```python
from build123d import *

# Parameters (mm, degrees)
F0_R     = 1.0414
F1_DEPTH = 12.7
F3_DEPTH = 25.4
F5_D     = 2.0828
F7_D     = 2.0828
F7_DEPTH = 15.24
F7_TIP   = 0.6257362487


with BuildPart() as f1:
    # F0 (on Top) → F1 (new body)
    with BuildSketch(Plane.XY):
        with BuildLine():
            ThreePointArc((-68.834, -11.2141), (-67.3461024484, -14.8062024484), (-63.754, -16.2941))
            Line((-63.754, -16.2941), (63.754, -16.2941))
            ThreePointArc((63.754, -16.2941), (67.3461024484, -14.8062024484), (68.834, -11.2141))
            Line((68.834, -11.2141), (68.834, 11.2141))
            ThreePointArc((68.834, 11.2141), (67.3461024484, 14.8062024484), (63.754, 16.2941))
            Line((63.754, 16.2941), (-63.754, 16.2941))
            ThreePointArc((-63.754, 16.2941), (-67.3461024484, 14.8062024484), (-68.834, 11.2141))
            Line((-68.834, 11.2141), (-68.834, -11.2141))
        make_face()
        with Locations((65.278, -10.16)):
            Circle(F0_R, mode=Mode.SUBTRACT)
        with Locations((65.278, 10.16)):
            Circle(F0_R, mode=Mode.SUBTRACT)
    extrude(amount=F1_DEPTH)

    # F2 (on face) → F3 (join)
    with BuildSketch(Plane.XY.offset(12.7)):
        with BuildLine():
            Line((-30.734, 16.2941), (-63.754, 16.2941))
            ThreePointArc((-63.754, 16.2941), (-67.3461024484, 14.8062024484), (-68.834, 11.2141))
            Line((-68.834, 11.2141), (-68.834, -11.2141))
            ThreePointArc((-68.834, -11.2141), (-67.3461024484, -14.8062024484), (-63.754, -16.2941))
            Line((-63.754, -16.2941), (-30.734, -16.2941))
            Line((-30.734, -16.2941), (-30.734, -6.35))
            ThreePointArc((-30.734, -6.35), (-37.084, 0), (-30.734, 6.35))
            Line((-30.734, 6.35), (-30.734, 16.2941))
        make_face()
    extrude(amount=F3_DEPTH)

    # F5 (through all)
    with Locations(Plane(origin=(-68.834, 0, 0), x_dir=(0, -1, 0), z_dir=(-1, 0, 0))):
        with Locations((-8.89, 33.02), (-8.89, 19.05), (8.89, 33.02), (8.89, 19.05)):
            Hole(F5_D / 2)

    # F7
    with Locations(Plane(origin=(0, 0, 0), x_dir=(1, 0, 0), z_dir=(0, 0, -1))):
        with Locations((-65.278, 10.16), (-65.278, -10.16)):
            Hole(F7_D / 2, depth=F7_DEPTH)
            with Locations((0, 0, -(F7_DEPTH + F7_TIP / 2))):  # 118° drill point
                Cone(0, F7_D / 2, F7_TIP, mode=Mode.SUBTRACT)


solid = f1.part
```
Could you check a few things on this model? Use its own coordinates, in mm. A direction names the side the tool comes from. Give positions to 0.01 mm unless a question says otherwise; leave off trailing zeros. Write each loop counter-clockwise with the first axis right and the second up, starting at its lowest first coordinate (ties: lowest second). Pieces come first, ordered by that corner, then holes. Notation, with made-up numbers: (-27, 82.5) - (-6, 82.5) arc R18 cw to (-6, 116.5) - close; hole circle Ø1 at (54, 84.5). An arc over 180 degrees is marked (long way). One line per item, written item: value. Start each with the question number.
Item 1: Imagine slicing it at A-A, the plane z = 27. List the corners of the cut face in (x, y) for me, and give its area (3 significant figures).
Item 2: I'm going to push flat-ended pins straight in: pin 1 (8 mm diameter, centred on x = -16, y = 9, fed in from -Z); pin 2 (1 mm diameter, centred on x = -20.5, y = 0.5, fed in from +Z); pin 3 (3.5 mm diameter, centred on y = -8.89, z = 19.05, fed in from +X); pin 4 (1.2 mm diameter, centred on y = 8.89, z = 19.05, fed in from +X). Where does each tip first touch, or does it pass through?
Item 3: Imagine slicing it at C-C, the plane x = -22. List the corners of the cut face in (y, z) for me, and give its area (3 significant figures).
Item 4: Which directions (+Z, -Z, +X, -X, +Y, -Y) give clear straight access to the entire face, cutting with the end or side of a thin tool? Please do faces 4 (the face through (-30.734, -11, 25)), 5 (the face through (-67.385, -14.766, 18.783)).
Item 5: Please list where these lines run through material, in increasing order: line 1 (Y direction, x = -43, z = 19); line 2 (Z direction, x = -43.5, y = 8.89); line 3 (X direction, y = -9.5, z = 5.5). Write a range as from..to.
Item 6: Imagine slicing it at B-B, the plane y = 0. List the corners of the cut face in (x, z) for me.
Item 7: Imagine slicing it at D-D, the plane y = -14. List the corners of the cut face in (x, z) for me, and give its area (3 significant figures).
Item 8: If we mould it in two halves opening along Y, with no side actions, what happens to faces 1 (the face through (-67.306, 14.845, 18.783)), 2 (the face through (-30.734, 11, 25)), 3 (the face through (-37.082, -0.14, 25.222))? For each: +Y half, -Y half, draft (parallel to the pull), parting line (faces both ways), or undercut.
Geometry says:
1. outline: (-68.83, -11.21) arc R5.08 ccw to (-63.75, -16.29) - (-30.73, -16.29) - (-30.73, -6.35) arc R6.35 cw to (-30.73, 6.35) - (-30.73, 16.29) - (-63.75, 16.29) arc R5.08 ccw to (-68.83, 11.21) - close
1. area: 1,170 mm^2
2. pin 1: z = 0
2. pin 2: z = 12.7
2. pin 3: x = -30.73
2. pin 4: through
3. outline: (-16.29, 0) - (16.29, 0) - (16.29, 12.7) - (-16.29, 12.7) - close
3. area: 414 mm^2
4. face 4: +Z, +X, +Y, -Y
4. face 5: +Z, -Z, -X, -Y
5. line 1: -16.29..-9.93, -7.85..7.85, 9.93..16.29
5. line 2: 0..18.01, 20.09..31.98, 34.06..38.1
5. line 3: -68.83..-66.08, -64.47..64.47, 66.08..68.83
6. outline: (-68.83, 0) - (68.83, 0) - (68.83, 12.7) - (-37.08, 12.7) - (-37.08, 38.1) - (-68.83, 38.1) - close
7. outline: (-68, 0) - (68, 0) - (68, 12.7) - (-30.73, 12.7) - (-30.73, 38.1) - (-68, 38.1) - close
7. area: 2,670 mm^2
8. face 1: +Y half
8. face 2: draft
8. face 3: undercut
